from build123d import *

# Parameters (mm, degrees)
BOX_W             = 10
BOX_H             = 10
BOX_DEPTH         = 10
SKETCH_W          = 4.4
SKETCH_H          = 4.4
PAD_DEPTH         = 4
PAD_FACE1_W       = 10
PAD_FACE1_H       = 10
POCKET_DEPTH      = 2.5
POCKET_FACE3_W    = 10
POCKET_FACE3_H    = 10
POCKET001_DEPTH   = 2.5
POCKET001_FACE6_W = 5
POCKET001_FACE6_H = 10
PAD001_DEPTH      = 10
SKETCH001_W       = 4.4
SKETCH001_H       = 4.4
PAD002_DEPTH      = 4
PAD002_FACE14_W   = 5
PAD002_FACE14_H   = 10
PAD003_DEPTH      = 10
SKETCH002_W       = 4.4
SKETCH002_H       = 4.4
PAD004_DEPTH      = 4
PAD004_FACE23_W   = 5
PAD004_FACE23_H   = 10
PAD005_DEPTH      = 10
SKETCH003_W       = 4.4
SKETCH003_H       = 4
PAD006_DEPTH      = 4
PAD006_FACE33_W   = 4.4
PAD006_FACE33_H   = 4
PAD007_DEPTH      = 0.4


with BuildPart() as part:
    # Box → Box (new body)
    with BuildSketch(Plane.XY):
        with Locations((5, 5)):
            Rectangle(BOX_W, BOX_H)
    extrude(amount=BOX_DEPTH)

    # Sketch (on Face6 of BaseFeature) → Pad (new body)
    with BuildSketch(Plane.XY.offset(10)):
        with Locations((5, 5)):
            Rectangle(SKETCH_W, SKETCH_H)
    extrude(amount=PAD_DEPTH)

    # Pad Face1 → Pocket (cut)
    with BuildSketch(Plane(origin=(0, 5, 5), x_dir=(0, 1, 0), z_dir=(-1, 0, 0))):
        Rectangle(PAD_FACE1_W, PAD_FACE1_H)
    extrude(amount=-POCKET_DEPTH, mode=Mode.SUBTRACT)

    # Pocket Face3 → Pocket001 (cut)
    with BuildSketch(Plane(origin=(10, 5, 5), x_dir=(0, -1, 0), z_dir=(1, 0, 0))):
        Rectangle(POCKET_FACE3_W, POCKET_FACE3_H)
    extrude(amount=-POCKET001_DEPTH, mode=Mode.SUBTRACT)

    # Pocket001 Face6 → Pad001 (add)
    with BuildSketch(Plane(origin=(5, 10, 5), x_dir=(1, 0, 0), z_dir=(0, 1, 0))):
        Rectangle(POCKET001_FACE6_W, POCKET001_FACE6_H)
    extrude(amount=PAD001_DEPTH)

    # Sketch001 (on Face8 of Pad001) → Pad002 (join)
    with BuildSketch(Plane.XY.offset(10)):
        with Locations((5, 15)):
            Rectangle(SKETCH001_W, SKETCH001_H)
    extrude(amount=PAD002_DEPTH)

    # Pad002 Face14 → Pad003 (add)
    with BuildSketch(Plane(origin=(5, 20, 5), x_dir=(1, 0, 0), z_dir=(0, 1, 0))):
        Rectangle(PAD002_FACE14_W, PAD002_FACE14_H)
    extrude(amount=PAD003_DEPTH)

    # Sketch002 (on Face16 of Pad003) → Pad004 (join)
    with BuildSketch(Plane.XY.offset(10)):
        with Locations((5, 25)):
            Rectangle(SKETCH002_W, SKETCH002_H)
    extrude(amount=PAD004_DEPTH)

    # Pad004 Face23 → Pad005 (add)
    with BuildSketch(Plane(origin=(5, 30, 5), x_dir=(1, 0, 0), z_dir=(0, 1, 0))):
        Rectangle(PAD004_FACE23_W, PAD004_FACE23_H)
    extrude(amount=PAD005_DEPTH)

    # Sketch003 (on Face25 of Pad005) → Pad006 (join)
    with BuildSketch(Plane.XY.offset(10)):
        with Locations((5, 34.8)):
            Rectangle(SKETCH003_W, SKETCH003_H)
    extrude(amount=PAD006_DEPTH)

    # Pad006 Face33 → Pad007 (add)
    with BuildSketch(Plane(origin=(5, 36.8, 12), x_dir=(1, 0, 0), z_dir=(0, 1, 0))):
        Rectangle(PAD006_FACE33_W, PAD006_FACE33_H)
    extrude(amount=PAD007_DEPTH)


solid = part.part
For this review, take the finished solid that the model builds, in its own axes (mm). A direction names the side the tool comes from. Give positions to 0.01 mm unless a question says otherwise; leave off trailing zeros. Order: outer loops, then holes, each group sorted by start corner. A loop starts at its lowest first (then second) coordinate and runs counter-clockwise, first axis right, second up. Notation, with made-up numbers: M 0,-33.75 L 9,-33.75 A14 cw 9,-13.75 Z; hole C 74,-1.5 d10. An arc over 180 degrees is marked long. Answer in a Markdown table with one row per item. Add a question column.
(1) Consider section A-A on z = 12.5. State the section outline as (x, y) points.
(2) For faces 1 (the face through (5, 17.2, 12)), 2 (the face through (7.2, 35, 12)), 3 (the face through (5, 35, 14)), 4 (the face through (2.8, 15, 12)), list the 3-axis set-ups (+Z, -Z, +X, -X, +Y, -Y) from which the entire face can be reached by the end or side of a thin tool; tool diameter is ignored.
(3) Consider section D-D on y = 11.5. State the section outline as (x, z) points.
(4) Wall thickness on probe 1 along Y at (x, z) = (3.85, 13); probe 2 along Z at (x, y) = (3.4, 8.5); probe 3 along X at (y, z) = (26.5, 13.25): over which ranges is each line inside the solid? List them lowest first. Write a range as [from, to].
(5) Mouldability with a two-part tool opening along Y and no side actions: class faces 5 (the face through (5, 27.2, 12)), 6 (the face through (5, 20, 0)), 7 (the face through (5, 2.8, 12)) as +Y half, -Y half, draft (parallel to the pull), parting line (faces both ways), or undercut.
(6) For pin 1 (3 mm diameter, centred on x = 4, z = 12.5, fed in from +Y); pin 2 (1.2 mm diameter, centred on y = 25, z = 13, fed in from -X); pin 3 (1.2 mm diameter, centred on x = 4.5, z = 11.5, fed in from -Y), all flat-tipped, find the tip position at first contact; note any pin that passes through.
(7) Consider section C-C on y = 34.5. State the section outline as (x, z) points.
(8) Consider section B-B on x = 6.45. State the section outline as (y, z) points.
Evaluation:
| question | item | result |
|---|---|---|
| 1 | outline | M 2.8,2.8 L 7.2,2.8 L 7.2,7.2 L 2.8,7.2 Z; M 2.8,12.8 L 7.2,12.8 L 7.2,17.2 L 2.8,17.2 Z; M 2.8,22.8 L 7.2,22.8 L 7.2,27.2 L 2.8,27.2 Z; M 2.8,32.8 L 7.2,32.8 L 7.2,37.2 L 2.8,37.2 Z |
| 2 | face 1 | +Z, +X, -X |
| 2 | face 2 | +Z, +X, +Y, -Y |
| 2 | face 3 | +Z, +X, -X, +Y, -Y |
| 2 | face 4 | +Z, -X, +Y, -Y |
| 3 | outline | M 2.5,0 L 7.5,0 L 7.5,10 L 2.5,10 Z |
| 4 | probe 1 | y = [2.8, 7.2], [12.8, 17.2], [22.8, 27.2], [32.8, 37.2] |
| 4 | probe 2 | z = [0, 10] |
| 4 | probe 3 | x = [2.8, 7.2] |
| 5 | face 5 | undercut |
| 5 | face 6 | draft |
| 5 | face 7 | -Y half |
| 6 | pin 1 | stops at y = 37.2 |
| 6 | pin 2 | stops at x = 2.8 |
| 6 | pin 3 | stops at y = 2.8 |
| 7 | outline | M 2.5,0 L 7.5,0 L 7.5,10 L 7.2,10 L 7.2,14 L 2.8,14 L 2.8,10 L 2.5,10 Z |
| 8 | outline | M 0,0 L 40,0 L 40,10 L 37.2,10 L 37.2,14 L 32.8,14 L 32.8,10 L 27.2,10 L 27.2,14 L 22.8,14 L 22.8,10 L 17.2,10 L 17.2,14 L 12.8,14 L 12.8,10 L 7.2,10 L 7.2,14 L 2.8,14 L 2.8,10 L 0,10 Z |
